Source: CAD feature listing. Evaluate the final solid. Frame: model axes, mm. A direction names the side the tool comes from. Coordinates: 2 decimals unless noted, no trailing zeros. Order: outer loops, then holes, each group sorted by start corner. A loop starts at its lowest first (then second) coordinate and runs counter-clockwise, first axis right, second up.
```python
from build123d import *

# Parameters (mm, degrees)
F1_DEPTH      = 16
F1_DEPTH_BACK = 16
F2_W          = 49.3
F2_H          = 1
F3_DEPTH      = 23.5
F3_DEPTH_BACK = 23.5
F5_SIZE       = 8
F6_DEPTH      = 5
F7_R          = 5
F8_R          = 1.75
F9_DEPTH      = 25


with BuildPart() as f1:
    # F0 (on Right) → F1 (new body, two sides)
    with BuildSketch(Plane.YZ) as f1_sk:
        Polygon((0, 20), (-1, 20), (-1, -15.8), (0, -14.8), align=None)
    extrude(amount=F1_DEPTH)
    extrude(f1_sk.sketch, amount=-F1_DEPTH_BACK)

    # F2 (on Right) → F3 (join, two sides)
    with BuildSketch(Plane.YZ) as f3_sk:
        with Locations((23.65, -15.3)):
            Rectangle(F2_W, F2_H)
    extrude(amount=F3_DEPTH)
    extrude(f3_sk.sketch, amount=-F3_DEPTH_BACK)

    # F5
    f5_edges = [f1.edges().sort_by_distance(p)[0] for p in [
        (-16, -0.5, 20),
        (16, -0.5, 20),
    ]]
    chamfer(f5_edges, length=F5_SIZE)

    # F4 (on Front) → F6 (cut)
    with BuildSketch(Plane.XZ):
        with BuildLine():
            Line((5, -5), (5, 5))
            ThreePointArc((5, 5), (0, 10), (-5, 5))
            Line((-5, 5), (-5, -5))
            ThreePointArc((-5, -5), (0, -10), (5, -5))
        make_face()
    extrude(amount=F6_DEPTH, mode=Mode.SUBTRACT)

    # F7
    f7_edges = [f1.edges().sort_by_distance(p)[0] for p in [
        (23.5, 48.3, -15.3),
        (-23.5, 48.3, -15.3),
        (23.5, -1, -15.3),
        (-23.5, -1, -15.3),
    ]]
    fillet(f7_edges, radius=F7_R)

    # F8 (on face) → F9 (cut)
    with BuildSketch(Plane.XY.offset(-14.8)):
        with Locations((-19.75, 44.55)):
            Circle(F8_R)
        with Locations((-19.75, 4.75)):
            Circle(F8_R)
        with Locations((19.75, 4.75)):
            Circle(F8_R)
        with Locations((19.75, 44.55)):
            Circle(F8_R)
    extrude(amount=-F9_DEPTH, mode=Mode.SUBTRACT)


solid = f1.part
```
Q1. Section query D-D on x = -13. Output: boundary loops of the cut face in (y, z).
Solutions:
outline: (-1, -15.8) - (48.3, -15.8) - (48.3, -14.8) - (0, -14.8) - (0, 15) - (-1, 15) - close
Q2. Pull-direction query (Y, two-part tool) for faces 4 (the flat face through (-12.1, -0.5, 15.9)), 5 (the cylindrical face through (-22.07, 46.8, -15.29)), 6 (the cylindrical face through (-21.14, 3.69, -15.29)); classes: pulls with the +Y half, pulls with the -Y half, needs draft (parallel to the pull), parting line crosses it, or undercut.
Solutions:
face 4: needs draft
face 5: pulls with the +Y half
face 6: undercut
Q3. Section query A-A on x = 0. Output: boundary loops of the cut face in (y, z), plus the area to 3 significant figures.
Solutions:
outline: (-1, -15.8) - (48.3, -15.8) - (48.3, -14.8) - (0, -14.8) - (0, -10) - (-1, -10) - close; (-1, 10) - (0, 10) - (0, 20) - (-1, 20) - close
area: 64.1 mm2
Q4. Set-up query: faces 1 (the cylindrical face through (-0.1, -0.5, -10)), 2 (the cylindrical face through (-22, 0.43, -15.29)), 3 (the flat face through (-7, 0, 2)). Return all of +Z, -Z, +X, -X, +Y, -Y with unobstructed straight access to the full face (end or side cutting, diameter ignored); none if empty.
Solutions:
face 1: +Y, -Y
face 2: +Z, -Z, -X, -Y
face 3: +Z, +X, -X, +Y
Q5. Section query C-C on z = 7.5. Output: boundary loops of the cut face in (x, y), plus the area to 3 significant figures.
Solutions:
outline: (-16, -1) - (-4.33, -1) - (-4.33, 0) - (-16, 0) - close; (4.33, -1) - (16, -1) - (16, 0) - (4.33, 0) - close
area: 23.3 mm2
Q6. Material intervals for line 1 along Y through (x, z) = (-19, -15); line 2 along X through (y, z) = (44, -15); line 3 along Z through (x, y) = (20, 10.5), sorted ascending.
Solutions:
line 1: y = -0.97 to 3.17, 6.33 to 42.97, 46.13 to 48.27
line 2: x = -23.45 to -21.41, -18.09 to 18.09, 21.41 to 23.45
line 3: z = -15.8 to -14.8
Q7. Section query B-B on y = 4.75. Output: boundary loops of the cut face in (x, z), plus the area to 3 significant figures.
Solutions:
outline: (-23.5, -15.8) - (-21.5, -15.8) - (-21.5, -14.8) - (-23.5, -14.8) - close; (-18, -15.8) - (18, -15.8) - (18, -14.8) - (-18, -14.8) - close; (21.5, -15.8) - (23.5, -15.8) - (23.5, -14.8) - (21.5, -14.8) - close
area: 40.0 mm2
Q8. Pin query (flat end, axial travel): P1, Ø0.5, axis at y = -0.5, z = 2, coming from the -X side; P2, Ø5.5, axis at x = -19.75, y = 44.55, coming from the +Z side; P3, Ø6, axis at x = 8, z = -5.5, coming from the +Y side; P4, Ø3, axis at x = -19.75, y = 4.75, coming from the -Z side (3 decimals). Return the tip coordinate at first contact, or that it passes through.
Solutions:
P1: stops at x = -16
P2: stops at z = -14.8
P3: stops at y = 0
P4: passes through
